Model file for the job. Use its own axes, mm. A direction names the side the tool comes from. Round coordinates to 2 decimals unless told otherwise and drop trailing zeros. Loops run counter-clockwise (first coordinate to the right, second up) from the corner with the lowest first, then second, coordinate; pieces in that order, holes last. Notation, with made-up numbers: M 36,77.5 L 47,77.5 A20 ccw 47,103.5 Z; hole C -38,59 d1. An arc over 180 degrees is marked long. Use a Markdown table: item, result. Add a question column.
Q1. Cut at B-B (z = 0). Give the cut face in (x, y), plus the area to 3 significant figures.
Q2. Pin check, flat tips, straight feed: pin 1 (3 mm diameter, centred on x = 28.5, z = -26.5, fed in from +Y); pin 2 (8 mm diameter, centred on y = 24, z = -19.5, fed in from +X); pin 3 (8 mm diameter, centred on x = 0, y = 30, fed in from +Z); pin 4 (8 mm diameter, centred on y = 25, z = 22, fed in from -X). Stop position of each tip, or through.
Q3. Probe line 1 (Z direction, x = -6, y = 36.5); line 2 (X direction, y = 4, z = 0); line 3 (Y direction, x = 0, z = 21). List the from-to ranges inside material, lowest first. Write a range as from..to.
Q4. Cut at A-A (y = 19). Give the cut face in (x, z), plus the area to 3 significant figures.
Q5. Mould opens along Z. For faces 1 (the face through (0, 23, 15)), 2 (the face through (0, 23, -15)), 3 (the face through (1.08, 25.12, -20.07)), 4 (the face through (4, 25, -25)) say: +Z half, -Z half, draft (parallel to the pull), parting line (faces both ways), or undercut.
Q6. Tool access for faces 5 (the face through (0.2, 6, 10.2)), 6 (the face through (20, 20, -20)), 7 (the face through (4, 25, 25)): list every direction of +Z, -Z, +X, -X, +Y, -Y with a clear straight run to the whole face (end or side of a thin tool).
Q7. Cut at D-D (x = -17). Give the cut face in (y, z).
from build123d import *

# Parameters (mm, degrees)
SKIZZE1_R                       = 60
AUFSATZ_LINEAR_AUSTRAGEN1_DEPTH = 10
SKIZZE2_W                       = 40
SKIZZE2_H                       = 10
AUFSATZ_LINEAR_AUSTRAGEN2_DEPTH = 40
VERRUNDUNG1_R                   = 20
SKIZZE3_R                       = 5
SCHNITT_LINEAR_AUSTRAGEN1_DEPTH = 116.433963806
SKIZZE4_R                       = 10
SCHNITT_LINEAR_AUSTRAGEN2_DEPTH = 10
SKIZZE5_R                       = 24
SCHNITT_LINEAR_AUSTRAGEN3_DEPTH = 30


with BuildPart() as part:
    # Skizze1 → Aufsatz-Linear austragen1 (new body)
    with BuildSketch(Plane(origin=(0, 0, 0), x_dir=(1, 0, 0), z_dir=(0, 1, 0))):
        with Locations(Location((0, 0, 0), (0, 0, 270))):
            Circle(SKIZZE1_R)
    extrude(amount=AUFSATZ_LINEAR_AUSTRAGEN1_DEPTH)

    # Skizze2 → Aufsatz-Linear austragen2 (add)
    with BuildSketch(Plane(origin=(0, 10, 0), x_dir=(1, 0, 0), z_dir=(0, 1, 0))):
        with Locations((0, -20)):
            Rectangle(SKIZZE2_W, SKIZZE2_H)
        with Locations((0, 20)):
            Rectangle(SKIZZE2_W, SKIZZE2_H)
    extrude(amount=AUFSATZ_LINEAR_AUSTRAGEN2_DEPTH)

    # Verrundung1
    verrundung1_edges = [part.edges().sort_by_distance(p)[0] for p in [
        (20, 50, -20),
        (20, 50, 20),
        (-20, 50, 20),
        (-20, 50, -20),
    ]]
    fillet(verrundung1_edges, radius=VERRUNDUNG1_R - 0.0001)  # a hair under: the kernel refuses the full size

    # Skizze3 → Schnitt-Linear austragen1 (cut, through all)
    with BuildSketch(Plane(origin=(0, 0, -25), x_dir=(-1, 0, 0), z_dir=(0, 0, -1))):
        with Locations((0, 30)):
            Circle(SKIZZE3_R)
    extrude(amount=-SCHNITT_LINEAR_AUSTRAGEN1_DEPTH, mode=Mode.SUBTRACT)

    # Skizze4 → Schnitt-Linear austragen2 (cut)
    with BuildSketch(Plane(origin=(0, 10, 0), x_dir=(1, 0, 0), z_dir=(0, 1, 0))):
        with Locations(Location((0, 0, 0), (0, 0, 270))):
            Circle(SKIZZE4_R)
    extrude(amount=-SCHNITT_LINEAR_AUSTRAGEN2_DEPTH, mode=Mode.SUBTRACT)

    # Skizze5 → Schnitt-Linear austragen3 (cut)
    with BuildSketch(Plane(origin=(0, 0, 15), x_dir=(-1, 0, 0), z_dir=(0, 0, -1))):
        with Locations((0, 30)):
            Circle(SKIZZE5_R)
    extrude(amount=SCHNITT_LINEAR_AUSTRAGEN3_DEPTH, mode=Mode.SUBTRACT)


solid = part.part
Checked values:
| question | item | result |
|---|---|---|
| 1 | outline | M -60,0 L -10,0 L -10,8.18 A24 cw -13.27,10 L -60,10 Z; M 10,0 L 60,0 L 60,10 L 13.27,10 A24 cw 10,8.18 Z |
| 1 | area | 994 mm^2 |
| 2 | pin 1 | stops at y = 10 |
| 2 | pin 2 | stops at x = 20 |
| 2 | pin 3 | passes through |
| 2 | pin 4 | stops at x = -20 |
| 3 | line 1 | z = -25..-15, 15..25 |
| 3 | line 2 | x = -60..-10, 10..60 |
| 3 | line 3 | y = 0..25, 35..50 |
| 4 | outline | M -20,-25 L 20,-25 L 20,-15 L -20,-15 Z; M -20,15 L 20,15 L 20,25 L -20,25 Z |
| 4 | area | 800 mm^2 |
| 5 | face 1 | undercut |
| 5 | face 2 | undercut |
| 5 | face 3 | draft |
| 5 | face 4 | -Z half |
| 6 | face 5 | +Y |
| 6 | face 6 | +Z, -Z, +X, +Y |
| 6 | face 7 | +Z, +X, -X, +Y |
| 7 | outline | M 0,-57.54 L 10,-57.54 L 10,-25 L 40.54,-25 L 40.54,-15 L 10,-15 L 10,15 L 40.54,15 L 40.54,25 L 10,25 L 10,57.54 L 0,57.54 Z |
